from build123d import *

# Parameters (mm, degrees)
SALIENTE_EXTRUIR1_DEPTH = 3
CORTAR_EXTRUIR1_DEPTH   = 3
CORTAR_EXTRUIR2_REACH   = 34.209
CROQUIS3_R              = 0.75
CROQUIS3_R_2            = 2.5


with BuildPart() as part:
    # Croquis1 → Saliente-Extruir1 (new body)
    with BuildSketch(Plane.XY):
        Polygon((-15, -28.345), (15, -28.345), (15, 28.345), (10, 28.345), (10, 25.345), (5, 25.345), (5, 28.345), (0, 28.345), (0, 25.345), (-5, 25.345), (-5, 28.345), (-10, 28.345), (-10, 25.345), (-15, 25.345), align=None)
    extrude(amount=SALIENTE_EXTRUIR1_DEPTH)

    # Croquis2 → Cortar-Extruir1 (cut)
    with BuildSketch(Plane(origin=(0, 0, 0), x_dir=(-1, 0, 0), z_dir=(0, 0, -1))):
        with BuildLine():
            Line((-15, -15.845), (-21.186751232, -15.845))
            Line((-21.186751232, -15.845), (-21.186751232, -34.648085908))
            Line((-21.186751232, -34.648085908), (21.188955731, -34.648085908))
            Line((21.188955731, -34.648085908), (21.188955731, -15.845))
            Line((21.188955731, -15.845), (15, -15.845))
            ThreePointArc((15, -15.845), (0, -30.845), (-15, -15.845))
        make_face()
    extrude(amount=-CORTAR_EXTRUIR1_DEPTH, mode=Mode.SUBTRACT)

    # Croquis3 → Cortar-Extruir2 (cut, up to next)
    with BuildSketch(Plane(origin=(0, 0, 0), x_dir=(-1, 0, 0), z_dir=(0, 0, -1)), mode=Mode.PRIVATE) as cortar_extruir2_sk1:
        with Locations((0, -10.845)):
            Circle(CROQUIS3_R)
    cortar_extruir2_tool1 = extrude(cortar_extruir2_sk1.sketch, amount=-CORTAR_EXTRUIR2_REACH, mode=Mode.PRIVATE) & part.part
    # Croquis3 → Cortar-Extruir2 (cut, up to next)
    with BuildSketch(Plane(origin=(0, 0, 0), x_dir=(-1, 0, 0), z_dir=(0, 0, -1)), mode=Mode.PRIVATE) as cortar_extruir2_sk2:
        with Locations((6.495190528, -14.595)):
            Circle(CROQUIS3_R)
    cortar_extruir2_tool2 = extrude(cortar_extruir2_sk2.sketch, amount=-CORTAR_EXTRUIR2_REACH, mode=Mode.PRIVATE) & part.part
    # Croquis3 → Cortar-Extruir2 (cut, up to next)
    with BuildSketch(Plane(origin=(0, 0, 0), x_dir=(-1, 0, 0), z_dir=(0, 0, -1)), mode=Mode.PRIVATE) as cortar_extruir2_sk3:
        with Locations((6.495190528, -22.095)):
            Circle(CROQUIS3_R)
    cortar_extruir2_tool3 = extrude(cortar_extruir2_sk3.sketch, amount=-CORTAR_EXTRUIR2_REACH, mode=Mode.PRIVATE) & part.part
    # Croquis3 → Cortar-Extruir2 (cut, up to next)
    with BuildSketch(Plane(origin=(0, 0, 0), x_dir=(-1, 0, 0), z_dir=(0, 0, -1)), mode=Mode.PRIVATE) as cortar_extruir2_sk4:
        with Locations((0, -25.845)):
            Circle(CROQUIS3_R)
    cortar_extruir2_tool4 = extrude(cortar_extruir2_sk4.sketch, amount=-CORTAR_EXTRUIR2_REACH, mode=Mode.PRIVATE) & part.part
    # Croquis3 → Cortar-Extruir2 (cut, up to next)
    with BuildSketch(Plane(origin=(0, 0, 0), x_dir=(-1, 0, 0), z_dir=(0, 0, -1)), mode=Mode.PRIVATE) as cortar_extruir2_sk5:
        with Locations((-6.495190528, -22.095)):
            Circle(CROQUIS3_R)
    cortar_extruir2_tool5 = extrude(cortar_extruir2_sk5.sketch, amount=-CORTAR_EXTRUIR2_REACH, mode=Mode.PRIVATE) & part.part
    # Croquis3 → Cortar-Extruir2 (cut, up to next)
    with BuildSketch(Plane(origin=(0, 0, 0), x_dir=(-1, 0, 0), z_dir=(0, 0, -1)), mode=Mode.PRIVATE) as cortar_extruir2_sk6:
        with Locations((-6.495190528, -14.595)):
            Circle(CROQUIS3_R)
    cortar_extruir2_tool6 = extrude(cortar_extruir2_sk6.sketch, amount=-CORTAR_EXTRUIR2_REACH, mode=Mode.PRIVATE) & part.part
    # Croquis3 → Cortar-Extruir2 (cut, up to next)
    with BuildSketch(Plane(origin=(0, 0, 0), x_dir=(-1, 0, 0), z_dir=(0, 0, -1)), mode=Mode.PRIVATE) as cortar_extruir2_sk7:
        with Locations((0, -18.345)):
            Circle(CROQUIS3_R_2)
    cortar_extruir2_tool7 = extrude(cortar_extruir2_sk7.sketch, amount=-CORTAR_EXTRUIR2_REACH, mode=Mode.PRIVATE) & part.part
    add(cortar_extruir2_tool1.solids().sort_by_distance((0, -10.845, 0))[0], mode=Mode.SUBTRACT)
    add(cortar_extruir2_tool2.solids().sort_by_distance((-6.495191, -14.595, 0))[0], mode=Mode.SUBTRACT)
    add(cortar_extruir2_tool3.solids().sort_by_distance((-6.495191, -22.095, 0))[0], mode=Mode.SUBTRACT)
    add(cortar_extruir2_tool4.solids().sort_by_distance((0, -25.845, 0))[0], mode=Mode.SUBTRACT)
    add(cortar_extruir2_tool5.solids().sort_by_distance((6.495191, -22.095, 0))[0], mode=Mode.SUBTRACT)
    add(cortar_extruir2_tool6.solids().sort_by_distance((6.495191, -14.595, 0))[0], mode=Mode.SUBTRACT)
    add(cortar_extruir2_tool7.solids().sort_by_distance((0, -18.345, 0))[0], mode=Mode.SUBTRACT)


solid = part.part
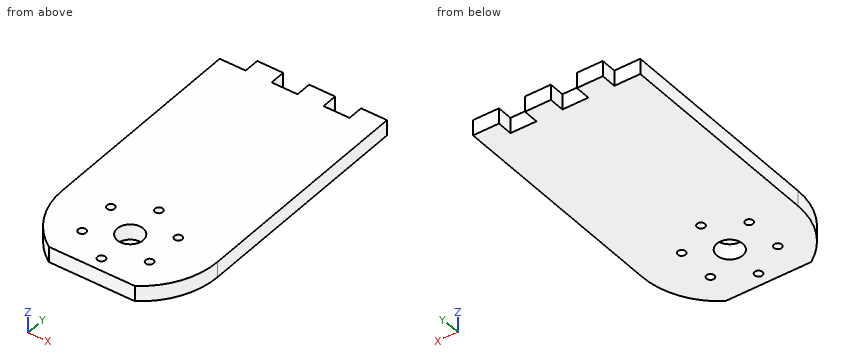
Build history of the part. All positions in model axes, mm. Coordinates: 2 decimals unless noted, no trailing zeros. Order: outer loops, then holes, each group sorted by start corner. A loop starts at its lowest first (then second) coordinate and runs counter-clockwise, first axis right, second up. Notation, with made-up numbers: (22, 25.5) - (27, 25.5) arc R19 ccw to (27, 41.5) - close; hole circle Ø10 at (-31, 66). An arc over 180 degrees is marked (long way). Write item = value, one per line. Start each with the question number.
1) Saw through at C-C on x = 10.75. Write the cut outline in (y, z) (3 decimals).
2) Saw through at B-B on z = 1. Write the cut outline in (x, y) (3 decimals).
3) Wall check: line 1 along Y through (x, z) = (6.5, 0.3) (3 decimals); line 2 along Y through (x, z) = (6, 2.25) (3 decimals); line 3 along Y through (x, z) = (-2.25, 1.4) (3 decimals). Give the ranges that are in metal, low to high. Write a range as from..to.
4) Flat gauge pins, fed straight in: pin 1 Ø1.5 at (x, z) = (-12, 1) entering from +Y (3 decimals); pin 2 Ø0.9 at (x, y) = (6.5, -14.6) entering from +Z. Where does each tip first touch, or does it go through?
5) Saw through at A-A on x = -1.5. Write the cut outline in (y, z) (3 decimals), then the cut area to 3 significant figures.
From the geometry:
q1.outline = (-26.306, 0) - (28.345, 0) - (28.345, 3) - (-26.306, 3) - close
q2.outline = (-15, -15.845) arc R15 ccw to (-8.292, -28.345) - (8.292, -28.345) arc R15 ccw to (15, -15.845) - (15, 28.345) - (10, 28.345) - (10, 25.345) - (5, 25.345) - (5, 28.345) - (0, 28.345) - (0, 25.345) - (-5, 25.345) - (-5, 28.345) - (-10, 28.345) - (-10, 25.345) - (-15, 25.345) - close; hole circle Ø1.5 at (-6.495, -22.095); hole circle Ø1.5 at (-6.495, -14.595); hole circle Ø5 at (0, -18.345); hole circle Ø1.5 at (0, -25.845); hole circle Ø1.5 at (0, -10.845); hole circle Ø1.5 at (6.495, -22.095); hole circle Ø1.5 at (6.495, -14.595)
q3.line_1 = -28.345..-22.845, -21.345..-15.345, -13.845..25.345
q3.line_2 = -28.345..-22.658, -21.532..-15.158, -14.032..25.345
q3.line_3 = -28.345..-19.435, -17.255..25.345
q4.pin_1 = 25.345
q4.pin_2 = through
q5.outline = (-28.345, 0) - (-20.345, 0) - (-20.345, 3) - (-28.345, 3) - close; (-16.345, 0) - (25.345, 0) - (25.345, 3) - (-16.345, 3) - close
q5.area = 149 mm^2
